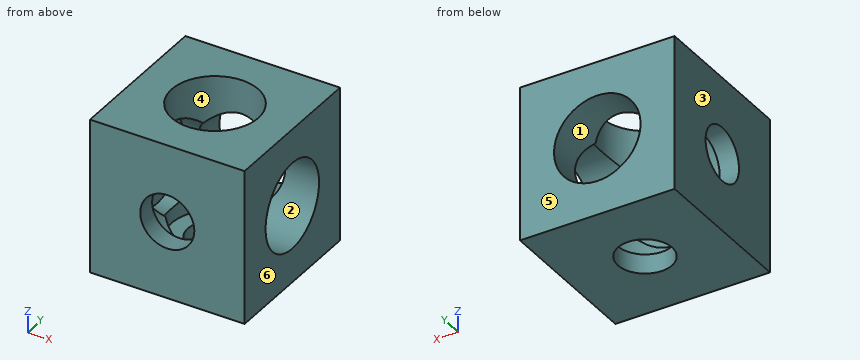
```python
from build123d import *

# Parameters (mm, degrees)
F0_W     = 20
F0_H     = 20
F0_R     = 5.6
F1_DEPTH = 20
F2_START = 17.5
F0_R_2   = 3.5
F2_DEPTH = 2.5
F3_R     = 5.6
F3_R_2   = 3.5
F4_DEPTH = 25
F5_START = -17.5
F5_DEPTH = 2.5
F6_R     = 5.6
F6_R_2   = 3.5
F7_DEPTH = 25
F8_START = -17.5
F8_DEPTH = 2.5


with BuildPart() as f1:
    # F0 (on Front) → F1 (new body)
    with BuildSketch(Plane.XZ):
        Rectangle(F0_W, F0_H)
        Circle(F0_R, mode=Mode.SUBTRACT)
    extrude(amount=F1_DEPTH)

    # F0 (on Front) → F2 (join)
    with BuildSketch(Plane.XZ.offset(F2_START)):
        Circle(F0_R)
        Circle(F0_R_2, mode=Mode.SUBTRACT)
    extrude(amount=F2_DEPTH)

    # F3 (on face) → F4 (cut)
    with BuildSketch(Plane.YZ.offset(10)):
        with Locations((-10, 0)):
            Circle(F3_R)
        with Locations((-10, 0)):
            Circle(F3_R_2, mode=Mode.SUBTRACT)
        with Locations((-10, 0)):
            Circle(F3_R_2)
    extrude(amount=-F4_DEPTH, mode=Mode.SUBTRACT)

    # F3 (on face) → F5 (join)
    with BuildSketch(Plane.YZ.offset(10).offset(F5_START)):
        with Locations((-10, 0)):
            Circle(F3_R)
        with Locations((-10, 0)):
            Circle(F3_R_2, mode=Mode.SUBTRACT)
    extrude(amount=-F5_DEPTH)

    # F6 (on face) → F7 (cut)
    with BuildSketch(Plane.XY.offset(10)):
        with Locations((0, -10)):
            Circle(F6_R)
        with Locations((0, -10)):
            Circle(F6_R_2, mode=Mode.SUBTRACT)
        with Locations((0, -10)):
            Circle(F6_R_2)
    extrude(amount=-F7_DEPTH, mode=Mode.SUBTRACT)

    # F6 (on face) → F8 (join)
    with BuildSketch(Plane.XY.offset(10).offset(F8_START)):
        with Locations((0, -10)):
            Circle(F6_R)
        with Locations((0, -10)):
            Circle(F6_R_2, mode=Mode.SUBTRACT)
    extrude(amount=-F8_DEPTH)


solid = f1.part
```
The model under review builds one solid part; all positions refer to its coordinate system, in mm. Face numbers are marked on the shaded views. A direction names the side the tool comes from. Round coordinates to 2 decimals unless told otherwise and drop trailing zeros. Loops run counter-clockwise (first coordinate to the right, second up) from the corner with the lowest first, then second, coordinate; pieces in that order, holes last. Notation, with made-up numbers: (-13, 68) -> (42, 68) arc R17 cw to (42, 76) -> close; hole circle Ø9 at (72.25, 56). An arc over 180 degrees is marked (long way). Answer in a Markdown table with one row per item.
1) Consider section B-B, the plane z = 0. Write out the cut boundary in (x, y).
Taken from the geometry:
| item | result |
|---|---|
| outline | (-10, -20) -> (-3.5, -20) -> (-3.5, -17.5) -> (-5.6, -17.5) -> (-5.6, -15.6) -> (-7.5, -15.6) -> (-7.5, -13.5) -> (-10, -13.5) -> close; (-10, -6.5) -> (-7.5, -6.5) -> (-7.5, -4.4) -> (-5.6, -4.4) -> (-5.6, 0) -> (-10, 0) -> close; (3.5, -20) -> (10, -20) -> (10, -15.6) -> (5.6, -15.6) -> (5.6, -17.5) -> (3.5, -17.5) -> close; (5.6, -4.4) -> (10, -4.4) -> (10, 0) -> (5.6, 0) -> close |
2) For pin 1 Ø9 at (y, z) = (-10, 0) entering from +X; pin 2 Ø8 at (x, z) = (0, 0) entering from +Y, all flat-tipped, find the tip position at first contact; note any pin that passes through.
Taken from the geometry:
| item | result |
|---|---|
| pin 1 | stops at x = -7.5 |
| pin 2 | stops at y = -17.5 |
3) Consider section A-A, the plane x = 0. Write out the cut boundary in (y, z).
Taken from the geometry:
| item | result |
|---|---|
| outline | (-20, -10) -> (-13.5, -10) -> (-13.5, -7.5) -> (-15.6, -7.5) -> (-15.6, -5.6) -> (-17.5, -5.6) -> (-17.5, -3.5) -> (-20, -3.5) -> close; (-20, 3.5) -> (-17.5, 3.5) -> (-17.5, 5.6) -> (-15.6, 5.6) -> (-15.6, 10) -> (-20, 10) -> close; (-6.5, -10) -> (0, -10) -> (0, -5.6) -> (-4.4, -5.6) -> (-4.4, -7.5) -> (-6.5, -7.5) -> close; (-4.4, 5.6) -> (0, 5.6) -> (0, 10) -> (-4.4, 10) -> close |
4) Consider section D-D, the plane y = -3.75. Write out the cut boundary in (x, z).
Taken from the geometry:
| item | result |
|---|---|
| outline | (-10, -10) -> (10, -10) -> (10, 10) -> (-10, 10) -> close; hole circle Ø11.2 at (0, 0) |
5) Consider section C-C, the plane z = 4.5. Write out the cut boundary in (x, y), plus the area to 3 significant figures.
Taken from the geometry:
| item | result |
|---|---|
| outline | (-10, -20) -> (10, -20) -> (10, -13.33) -> (4.5, -13.33) arc R5.6 cw to (3.33, -14.5) -> (3.33, -17.5) -> (-3.33, -17.5) -> (-3.33, -14.5) arc R5.6 cw to (-4.5, -13.33) -> (-7.5, -13.33) -> (-7.5, -6.67) -> (-4.5, -6.67) arc R5.6 cw to (-3.33, -5.5) -> (-3.33, 0) -> (-10, 0) -> close; (3.33, -5.5) arc R5.6 cw to (4.5, -6.67) -> (10, -6.67) -> (10, 0) -> (3.33, 0) -> close |
| area | 208 mm² |
6) Draft analysis for pull direction X (two halves, no side actions). For the marked faces 4, 5 and 6, state which applies: pulls with the +X half, pulls with the -X half, needs draft (parallel to the pull), parting line crosses it, or undercut.
Taken from the geometry:
| item | result |
|---|---|
| face 4 | undercut |
| face 5 | needs draft |
| face 6 | pulls with the +X half |
7) Wall thickness on line 1 along X through (y, z) = (-2.5, 0); line 2 along Z through (x, y) = (0.75, -5.25): over which ranges is each line inside the solid? List them lowest first.
Taken from the geometry:
| item | result |
|---|---|
| line 1 | x = -10 to -5.6, 5.6 to 10 |
| line 2 | z = -10 to -7.5 |
8) Tool access review of the marked faces 1, 2 and 3: name each direction out of +Z, -Z, +X, -X, +Y, -Y from which nothing blocks a thin tool from reaching the whole face with its end or side.
Taken from the geometry:
| item | result |
|---|---|
| face 1 | +Y |
| face 2 | +X |
| face 3 | +Z, -Z, -X, +Y, -Y |
